from build123d import *

# Parameters (mm, degrees)
SKETCH1_W           = 80
SKETCH1_H           = 110
BOSS_EXTRUDE1_DEPTH = 80
SKETCH2_W           = 50
SKETCH2_H           = 110
CUT_EXTRUDE2_DEPTH  = 47
SKETCH3_R           = 4
CUT_EXTRUDE3_DEPTH  = 81


with BuildPart() as part:
    # Sketch1 → Boss-Extrude1 (new body)
    with BuildSketch(Plane(origin=(0, 0, 0), x_dir=(1, 0, 0), z_dir=(0, 1, 0))):
        with Locations((10.955882353, 0.606617647)):
            Rectangle(SKETCH1_W, SKETCH1_H)
    extrude(amount=BOSS_EXTRUDE1_DEPTH)

    # Sketch2 → Cut-Extrude2 (cut)
    with BuildSketch(Plane(origin=(0, 80, 0), x_dir=(1, 0, 0), z_dir=(0, 1, 0))):
        with Locations((25.955882353, 0.606617647)):
            Rectangle(SKETCH2_W, SKETCH2_H)
    extrude(amount=-CUT_EXTRUDE2_DEPTH, mode=Mode.SUBTRACT)

    # Sketch3 → Cut-Extrude3 (cut, through all)
    with BuildSketch(Plane.ZY.offset(29.044117647)):
        with Locations((41.893382353, 67.5)):
            Circle(SKETCH3_R)
        with Locations((-43.106617647, 67.5)):
            Circle(SKETCH3_R)
    extrude(amount=-CUT_EXTRUDE3_DEPTH, mode=Mode.SUBTRACT)


solid = part.part
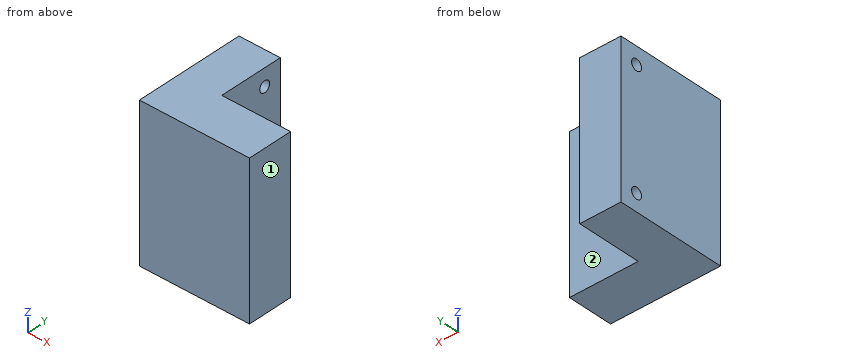
Geometry check sheet. Reference: the model listing, model coordinates, mm. Face numbers are marked on the shaded views. A direction names the side the tool comes from. Round coordinates to 2 decimals unless told otherwise and drop trailing zeros. Loops run counter-clockwise (first coordinate to the right, second up) from the corner with the lowest first, then second, coordinate; pieces in that order, holes last. Notation, with made-up numbers: (-13, 73.5) - (8, 73.5) arc R12 cw to (8, 92.5) - close; hole circle Ø6 at (37, -29.5). An arc over 180 degrees is marked (long way). One line per question, with ' | ' between items. Start each with the question number.
1. Cross-section at B-B on z = 4. Record the cut outline in (x, y).
2. Tool access check on the marked faces 1 and 2. Record the directions out of +Z, -Z, +X, -X, +Y, -Y that give a thin tool (end or side, any length) a straight path to the whole face; none if there is none.
3. Cross-section at D-D on y = 53.5. Record the cut outline in (x, z), then the cut area to 3 significant figures.
4. Cross-section at C-C on x = 20.5. Record the cut outline in (y, z), then the cut area to 3 significant figures.
5. Depth check by flat-ended pin: pin 1 (23.5 mm diameter, centred on y = 62, z = -15.5, fed in from +X); pin 2 (12 mm diameter, centred on x = 33.5, z = -2.5, fed in from +Y). Enter the tip coordinate at first touch or a pass-through.
6. Scan lines: line 1 (Z direction, x = -23, y = 67); line 2 (X direction, y = 63, z = -9); line 3 (Y direction, x = 33.5, z = -21.5). Record each from-to range of solid material in increasing order. Write a range as [from, to].
7. Cross-section at A-A on y = 67.5. Record the cut outline in (x, z), then the cut area to 3 significant figures.
Taken from the geometry:
1) outline: (-29.04, 0) - (50.96, 0) - (50.96, 33) - (0.96, 33) - (0.96, 80) - (-29.04, 80) - close
2) face 1: +Z, -Z, +X, +Y, -Y | face 2: +Z, -Z, +X, +Y
3) outline: (-29.04, -55.61) - (0.96, -55.61) - (0.96, 54.39) - (-29.04, 54.39) - close | area: 3,300 mm²
4) outline: (0, -55.61) - (33, -55.61) - (33, 54.39) - (0, 54.39) - close | area: 3,630 mm²
5) pin 1: x = 0.96 | pin 2: y = 33
6) line 1: [-55.61, -47.08], [-39.14, 37.92], [45.86, 54.39] | line 2: [-29.04, 0.96] | line 3: [0, 33]
7) outline: (-29.04, -55.61) - (0.96, -55.61) - (0.96, -47.11) - (-29.04, -47.11) - close; (-29.04, -39.11) - (0.96, -39.11) - (0.96, 37.89) - (-29.04, 37.89) - close; (-29.04, 45.89) - (0.96, 45.89) - (0.96, 54.39) - (-29.04, 54.39) - close | area: 2,820 mm²
